Geometry: see drawing. Coordinates: mm, zero at the bounding-box minimum. A direction names the side the tool comes from. Coordinates: 2 decimals unless noted, no trailing zeros. Loops run counter-clockwise (first coordinate to the right, second up) from the corner with the lowest first, then second, coordinate; pieces in that order, holes last. Notation, with made-up numbers: M 46.5,-37.75 L 73.5,-37.75 A15 cw 73.5,-15.75 Z; hole C 29.25,-38.5 d2. An arc over 180 degrees is marked long. Write each question's results on one line, items separated by ' | '. Start each with the question number.
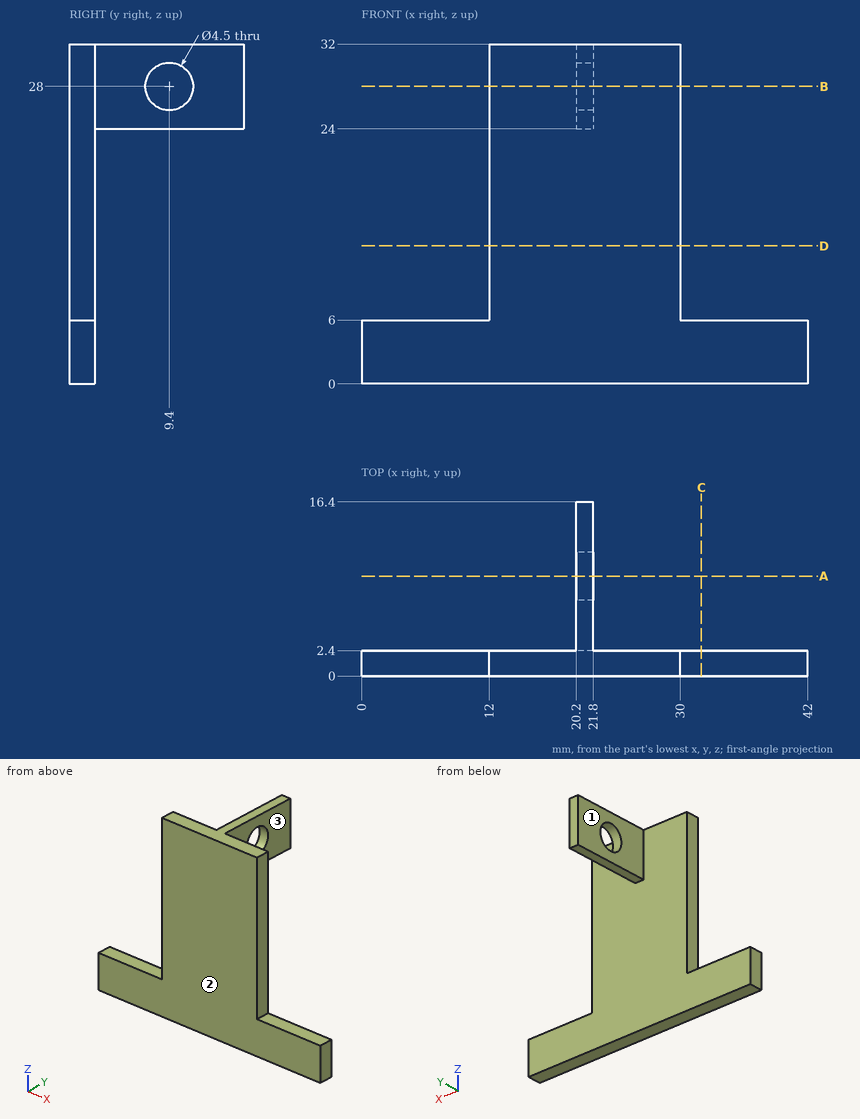
Item 1: Cut plane A-A (y = 9.4). Output: boundary loops of the cut face in (x, z), then the cut area to 3 significant figures.
Item 2: First-contact query: pin 1 Ø6 at (x, z) = (31, 27) entering from +Y; pin 2 Ø1.9 at (x, y) = (36.5, 1.5) entering from +Z; pin 3 Ø1 at (y, z) = (3, 28.5) entering from +X. Flat tips, straight axial feed; report the tip coordinate or a pass-through.
Item 3: Access query for the marked faces 1, 2 and 3. Directions: +Z, -Z, +X, -X, +Y, -Y. A direction counts if a zero-diameter tool reaches every point of the face in a straight line with its end or side. Return the directions, or none.
Item 4: Cut plane C-C (x = 32). Output: boundary loops of the cut face in (y, z), then the cut area to 3 significant figures.
Item 5: Cut plane D-D (z = 13). Output: boundary loops of the cut face in (x, y), then the cut area to 3 significant figures.
Item 6: Cut plane B-B (z = 28). Output: boundary loops of the cut face in (x, y), then the cut area to 3 significant figures.
Item 7: Line query: probe 1 along Y at (x, z) = (20.8, 28); probe 2 along X at (y, z) = (1, 28); probe 3 along Y at (x, z) = (19.5, 23). Output: solid intervals per line, ascending.
Response values:
1) outline: M 20.2,24 L 21.8,24 L 21.8,25.75 L 20.2,25.75 Z; M 20.2,30.25 L 21.8,30.25 L 21.8,32 L 20.2,32 Z | area: 5.60 mm2
2) pin 1: stops at y = 2.4 | pin 2: stops at z = 6 | pin 3: stops at x = 21.8
3) face 1: +Z, -Z, -X, +Y | face 2: +Z, -Z, +X, -X, -Y | face 3: +Z, -Z, +X, +Y
4) outline: M 0,0 L 2.4,0 L 2.4,6 L 0,6 Z | area: 14.4 mm2
5) outline: M 12,0 L 30,0 L 30,2.4 L 12,2.4 Z | area: 43.2 mm2
6) outline: M 12,0 L 30,0 L 30,2.4 L 21.8,2.4 L 21.8,7.15 L 20.2,7.15 L 20.2,2.4 L 12,2.4 Z; M 20.2,11.65 L 21.8,11.65 L 21.8,16.4 L 20.2,16.4 Z | area: 58.4 mm2
7) probe 1: y = 0 to 7.15, 11.65 to 16.4 | probe 2: x = 12 to 30 | probe 3: y = 0 to 2.4
